from build123d import *

# Parameters (mm, degrees)
F0_R     = 12.5
F1_DEPTH = 10


with BuildPart() as f1:
    # F0 (on Top) → F1 (new body)
    with BuildSketch(Plane.XY):
        with BuildLine():
            ThreePointArc((0, 17.5), (5.125631, 5.125631), (17.5, 0))
            Line((17.5, 0), (95, 0))
            ThreePointArc((95, 0), (98.535534, 1.464466), (100, 5))
            Line((100, 5), (100, 30))
            ThreePointArc((100, 30), (98.535534, 33.535534), (95, 35))
            Line((95, 35), (17.5, 35))
            ThreePointArc((17.5, 35), (5.125631, 29.874369), (0, 17.5))
        make_face()
        with Locations((17.5, 17.5)):
            Circle(F0_R, mode=Mode.SUBTRACT)
    extrude(amount=F1_DEPTH)


solid = f1.part
Read the model definition and answer for the solid it produces. Units are mm, in the model's axes. Coordinates: 2 decimals unless noted, no trailing zeros. Write each loop counter-clockwise with the first axis right and the second up, starting at its lowest first coordinate (ties: lowest second). Pieces come first, ordered by that corner, then holes. Notation, with made-up numbers: (-30.5, 18.5) -> (8.5, 18.5) arc R14 cw to (8.5, 32.5) -> close; hole circle Ø9 at (-12, -34). An arc over 180 degrees is marked (long way). Return JSON: item names as keys, results as strings.
(1) For a pull along X with two mould halves and no side action, classify faces 1 (the cylindrical face through (99, 33, 5)), 2 (the flat face through (60, 18, 0)), 3 (the cylindrical face through (14.79, 5.297, 4.93)) as pulls with the +X half, pulls with the -X half, needs draft (parallel to the pull), parting line crosses it, or undercut.
Answers below:
{"face 1": "pulls with the +X half", "face 2": "needs draft", "face 3": "undercut"}
(2) The part is cut by section A-A on z = 7.5. Give the vertices of the cut face in (x, y), then the cut area to 3 significant figures.
Answers below:
{"outline": "(0, 17.5) arc R17.5 ccw to (17.5, 0) -> (95, 0) arc R5 ccw to (100, 5) -> (100, 30) arc R5 ccw to (95, 35) -> (17.5, 35) arc R17.5 ccw to start; hole circle Ø25 at (17.5, 17.5)", "area": "2,870 mm^2"}
(3) The part is cut by section B-B on y = 8.5. Give the vertices of the cut face in (x, z).
Answers below:
{"outline": "(2.49, 0) -> (8.83, 0) -> (8.83, 10) -> (2.49, 10) -> close; (26.17, 0) -> (100, 0) -> (100, 10) -> (26.17, 10) -> close"}
(4) Consider line 1 along Y through (x, z) = (17.5, 5.75); line 2 along X through (y, z) = (17, 1.25); line 3 along Y through (x, z) = (29, 1). Determine where each line is inside the solid, lowest interval first. Write a range as from..to.
Answers below:
{"line 1": "0..5, 30..35", "line 2": "0.01..5.01, 29.99..100", "line 3": "0..12.6, 22.4..35"}
